Work out the finished part from the listing and answer in its coordinate system (mm). Face numbers are marked on the shaded views. Coordinates: 2 decimals unless noted, no trailing zeros. Loops run counter-clockwise (first coordinate to the right, second up) from the corner with the lowest first, then second, coordinate; pieces in that order, holes last. Notation, with made-up numbers: (25.5, -21.5) - (36.5, -21.5) arc R20 ccw to (36.5, -9.5) - close; hole circle Ø8 at (60, 21.5). An arc over 180 degrees is marked (long way). Write each question's results on one line, items separated by ' | '. Start each with the question number.
Item 1: Section C-C, the plane x = 45 is taken. Write down the section's boundary in (y, z), plus the area to 3 significant figures.
Item 2: Each of these flat-tipped pins is pushed along its axis until it touches: pin 1 Ø2 at (x, y) = (31, 15) entering from +Z; pin 2 Ø5 at (x, y) = (74, 41) entering from -Z. Where does it stop, or does it pass through?
Item 3: Section D-D, the plane x = 87 is taken. Write down the section's boundary in (y, z).
Item 4: Consider probe 1 along Y at (x, z) = (3, 2.8); probe 2 along Y at (x, z) = (12.5, 5.1); probe 3 along X at (y, z) = (16.5, 2.75). Determine where each line is inside the solid, lowest interval first. Write a range as [from, to].
Item 5: For a pull along X with two mould halves and no side action, classify the marked faces 1 and 2 as +X half, -X half, draft (parallel to the pull), parting line (faces both ways), or undercut.
Item 6: Section B-B, the plane z = 2.05 is taken. Write down the section's boundary in (x, y), plus the area to 3 significant figures.
Item 7: Section A-A, the plane y = 41 is taken. Write down the section's boundary in (x, z).
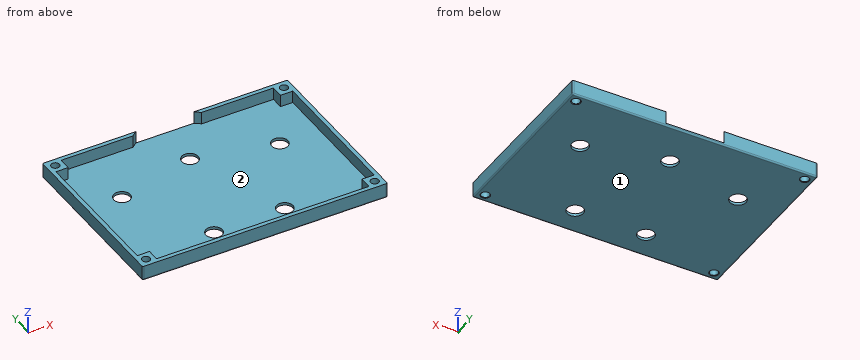
from build123d import *

# Parameters (mm, degrees)
F0_W      = 90
F0_H      = 64
F1_DEPTH  = 1
F3_W      = 90
F3_H      = 64
F3_W_2    = 87
F3_H_2    = 61
F4_DEPTH  = 4.5
F5_R      = 3
F6_DEPTH  = 1.001
F8_DEPTH  = 4.501
F10_W     = 4.5
F10_H     = 4.5
F11_DEPTH = 4.5
F12_R     = 1.5
F13_DEPTH = 5.501
F14_R     = 0.5
F16_SIZE  = 0.2


# Not quite as in the source:
# - two fillets or chamfers of one size are made in one step


with BuildPart() as f1:
    # F0 (on Top) → F1 (new body)
    with BuildSketch(Plane.XY):
        with Locations((45, 32)):
            Rectangle(F0_W, F0_H)
    extrude(amount=F1_DEPTH)

    # F3 (on face) → F4 (join)
    with BuildSketch(Plane.XY.offset(1)):
        with Locations((45, 32)):
            Rectangle(F3_W, F3_H)
        with Locations((45, 32)):
            Rectangle(F3_W_2, F3_H_2, mode=Mode.SUBTRACT)
    extrude(amount=F4_DEPTH)

    # F5 (on face) → F6 (cut, through all)
    with BuildSketch(Plane.XY.offset(1)):
        with Locations((16, 41)):
            Circle(F5_R)
        with Locations((45, 48)):
            Circle(F5_R)
        with Locations((32, 10)):
            Circle(F5_R)
        with Locations((58, 10)):
            Circle(F5_R)
        with Locations((74, 41)):
            Circle(F5_R)
    extrude(amount=-F6_DEPTH, mode=Mode.SUBTRACT)

    # F7 (on face) → F8 (cut, through all)
    with BuildSketch(Plane.XY.offset(1)):
        with BuildLine():
            ThreePointArc((34.3868006709, 64), (35.920722141, 31.0823549641), (64.2, 48))
            ThreePointArc((64.2, 48), (61.9176450359, 57.079277859), (55.6131993291, 64))
            Line((55.6131993291, 64), (34.3868006709, 64))
        make_face()
    extrude(amount=F8_DEPTH, mode=Mode.SUBTRACT)

    # F10 (on face) → F11 (join, through all)
    with BuildSketch(Plane.XY.offset(1)):
        with Locations((86.25, 3.75)):
            Rectangle(F10_W, F10_H)
        with Locations((86.25, 60.25)):
            Rectangle(F10_W, F10_H)
        with Locations((3.75, 3.75)):
            Rectangle(F10_W, F10_H)
        with Locations((3.75, 60.25)):
            Rectangle(F10_W, F10_H)
    extrude(amount=F11_DEPTH)

    # F12 (on face) → F13 (cut, through all)
    with BuildSketch(Plane.XY.offset(5.5)):
        with Locations((87, 3)):
            Circle(F12_R)
        with Locations((3, 3)):
            Circle(F12_R)
        with Locations((87, 61)):
            Circle(F12_R)
        with Locations((3, 61)):
            Circle(F12_R)
    extrude(amount=-F13_DEPTH, mode=Mode.SUBTRACT)

    # F14
    f14_edges = [f1.edges().sort_by_distance(p)[0] for p in [
        (45, 64, 0),
        (0, 64, 2.75),
        (0, 0, 2.75),
        (0, 32, 0),
        (90, 64, 2.75),
        (90, 0, 2.75),
        (45, 0, 0),
        (90, 32, 0),
    ]]
    fillet(f14_edges, radius=F14_R)

    # F16
    f16_edges = [f1.edges().sort_by_distance(p)[0] for p in [
        (85.5, 61, 0),
        (85.5, 3, 0),
        (1.5, 3, 0),
        (1.5, 61, 0),
    ]]
    chamfer(f16_edges, length=F16_SIZE)


solid = f1.part
Answer key:
1) outline: (0, 0.5) arc R0.5 ccw to (0.5, 0) - (45, 0) - (45, 1) - (1.5, 1) - (1.5, 5.5) - (0, 5.5) - close; (51, 0) - (63.5, 0) arc R0.5 ccw to (64, 0.5) - (64, 1) - (51, 1) - close | area: 64.6 mm^2
2) pin 1: stops at z = 1 | pin 2: passes through
3) outline: (0, 0.5) arc R0.5 ccw to (0.5, 0) - (1.3, 0) - (1.5, 0.2) - (1.5, 5.5) - (0, 5.5) - close; (4.5, 0.2) - (4.7, 0) - (59.3, 0) - (59.5, 0.2) - (59.5, 5.5) - (58, 5.5) - (58, 1) - (6, 1) - (6, 5.5) - (4.5, 5.5) - close; (62.5, 0.2) - (62.7, 0) - (63.5, 0) arc R0.5 ccw to (64, 0.5) - (64, 5.5) - (62.5, 5.5) - close
4) probe 1: y = [0, 1.5], [4.5, 6], [58, 59.5], [62.5, 64] | probe 2: y = [0, 1.5], [62.5, 64] | probe 3: x = [0, 1.5], [88.5, 90]
5) face 1: draft | face 2: undercut
6) outline: (0, 0.5) arc R0.5 ccw to (0.5, 0) - (89.5, 0) arc R0.5 ccw to (90, 0.5) - (90, 63.5) arc R0.5 ccw to (89.5, 64) - (55.61, 64) arc R19.2 cw to (57.59, 62.5) - (84, 62.5) - (84, 58) - (88.5, 58) - (88.5, 6) - (84, 6) - (84, 1.5) - (6, 1.5) - (6, 6) - (1.5, 6) - (1.5, 58) - (6, 58) - (6, 62.5) - (32.41, 62.5) arc R19.2 cw to (34.39, 64) - (0.5, 64) arc R0.5 ccw to (0, 63.5) - close; hole circle Ø3 at (3, 3); hole circle Ø3 at (3, 61); hole circle Ø3 at (87, 3); hole circle Ø3 at (87, 61) | area: 471 mm^2
7) outline: (0, 0.5) arc R0.5 ccw to (0.5, 0) - (13, 0) - (13, 1) - (1.5, 1) - (1.5, 5.5) - (0, 5.5) - close; (19, 0) - (71, 0) - (71, 1) - (19, 1) - close; (77, 0) - (89.5, 0) arc R0.5 ccw to (90, 0.5) - (90, 5.5) - (88.5, 5.5) - (88.5, 1) - (77, 1) - close
